Autodesk Inventor part; units mm, degrees
ref_plane "YZ Plane" through (0, 0, 0) normal (1, 0, 0) x (0, 1, 0)
ref_plane "XZ Plane" through (0, 0, 0) normal (0, 1, 0) x (-1, 0, 0)
ref_plane "XY Plane" through (0, 0, 0) normal (0, 0, 1) x (1, 0, 0)
sketch "Sketch1" plane through (0, 0, 0) normal (0, 0, 1) x (1, 0, 0)
  line L0 (5.9771, 0) -> (28.2021, 0)
  line L1 (28.2021, 0) -> (28.2021, 3.175)
  line L2 (28.2021, 3.175) -> (5.9771, 3.175)
  line L3 (2.8021, 6.35) -> (2.8021, 25.4)
  line L4 (5.9771, 28.575) -> (28.2021, 28.575)
  line L5 (28.2021, 28.575) -> (28.2021, 31.75)
  line L6 (28.2021, 31.75) -> (5.9771, 31.75)
  line L7 (-0.3729, 25.4) -> (-0.3729, 6.35)
  arc A0 (5.9771, 28.575) -> (2.8021, 25.4) centre (5.9771, 25.4) ccw
  arc A1 (2.8021, 6.35) -> (5.9771, 3.175) centre (5.9771, 6.35) ccw
  arc A2 (5.9771, 31.75) -> (-0.3729, 25.4) centre (5.9771, 25.4) ccw
  arc A3 (-0.3729, 6.35) -> (5.9771, 0) centre (5.9771, 6.35) ccw
  point P0 (0, 0)
  point P1 (-0.3729, 0)
  point P2 (2.8021, 3.175)
  point P3 (2.8021, 28.575)
  dimension "d0" = 28.575
  dimension "d1" = 3.175
  dimension "d2" = 25.4
  dimension "d3" = 25.4
  dimension "d4" = 3.175
  dimension "d5" = 3.175
  dimension "d6" = 6.35
extrude "Extrusion1" add sketch "Sketch1" against normal blind 889
sketch "Sketch2" plane through (-0.3729, 6.35, 0) normal (-1, 0, 0) x (0, 0, 1)
  line L0 (0, 19.05) -> (-889, 19.05)
  line L1 (-228.6, 0) -> (-228.6, 7.9375)
  arc A0 (-228.6, 11.1125) -> (-228.6, 7.9375) centre (-228.6, 9.525) ccw
  line L2 (-228.6, 11.1125) -> (-228.6, 19.05)
  line L3 (-228.6, 19.05) -> (-889, 19.05)
  line L4 (-889, 0) -> (-889, 19.05)
  line L5 (-889, 0) -> (-228.6, 0)
  circle A1 centre (-552.45, 11.43) radius 4.826
  circle A2 centre (-501.65, 11.43) radius 4.826
  circle A3 centre (-387.35, 11.43) radius 4.826
  circle A4 centre (-336.55, 11.43) radius 4.826
  circle A5 centre (-444.5, 7.62) radius 4.826
  circle A6 centre (-730.25, 11.43) radius 4.826
  circle A7 centre (-781.05, 11.43) radius 4.826
  line L6 (0, 25.4) -> (-889, 25.4) construction
  circle A8 centre (-133.35, 11.43) radius 4.826
  circle A9 centre (-82.55, 11.43) radius 4.826
  point P0 (0, -6.35)
  point P1 (-254, 0.852)
  dimension "d10" = 7.62
  dimension "d11" = 3.81
  dimension "d14" = 254
hole "Hole1" at (-0.3729, 17.78, -781.05) at (-0.3729, 17.78, -730.25) at (-0.3729, 17.78, -552.45) at (-0.3729, 17.78, -501.65) at (-0.3729, 13.97, -444.5) at (-0.3729, 17.78, -387.35) at (-0.3729, 17.78, -336.55) at (-0.3729, 17.78, -133.35) at (-0.3729, 17.78, -82.55) direction (1, 0, 0) diameter 9.652 end through all
hole "Hole2" at (-0.3729, 15.875, -228.6) direction (1, 0, 0) diameter 3.175 end through all
sketch "Sketch3" plane through (5.9771, 31.75, 0) normal (0, 1, 0) x (1, 0, 0)
  line L0 (22.225, 889) -> (0, 889)
  line L1 (22.225, 0) -> (22.225, 889)
  point P0 (-5.9771, 0)
  point P1 (9.525, 876.3)
  dimension "d34" = 12.7
  dimension "d35" = 12.7
hole "Hole3" at (15.5021, 31.75, -876.3) direction (0, -1, 0) diameter 6.5278 end through all
pattern_linear "Rectangular Pattern1" count 35 spacing 25.4 along (0, 0, 1) of "Hole3"
sketch "Sketch4" plane through (5.9771, 31.75, 0) normal (0, 1, 0) x (1, 0, 0)
  circle A0 centre (9.525, 12.7) radius 3.2639
  circle A1 centre (9.525, 38.1) radius 3.2639
  circle A2 centre (9.525, 63.5) radius 3.2639
  circle A3 centre (9.525, 88.9) radius 3.2639
  circle A4 centre (9.525, 114.3) radius 3.2639
  circle A5 centre (9.525, 139.7) radius 3.2639
  circle A6 centre (9.525, 165.1) radius 3.2639
  circle A7 centre (9.525, 190.5) radius 3.2639
  line L0 (22.225, 0) -> (-13.6032, 0)
  line L1 (-13.6032, 0) -> (-13.6032, 508)
  line L2 (-13.6032, 508) -> (22.225, 508)
  line L3 (22.225, 508) -> (22.225, 0)
  point P0 (-5.9771, 0)
  dimension "d46" = 508
extrude "Extrusion2" cut sketch "Sketch4" against normal blind 38.1
properties part number "chassis 15 inch"
Could you check a few things on this model? Use its own coordinates, in mm. A direction names the side the tool comes from. Give positions to 0.01 mm unless a question says otherwise; leave off trailing zeros. Order: outer loops, then holes, each group sorted by start corner. A loop starts at its lowest first (then second) coordinate and runs counter-clockwise, first axis right, second up.
1. Suppose I cut it at B-B (z = -800.1). List the corners of the cut face in (x, y) for me (3 decimals), plus the area to 3 significant figures.
2. Will these pins go through, and if not, where does the flat tip stop? P1, Ø8.5, axis at x = 15.5, z = -774.7, coming from the -Y side; P2, Ø1.5, axis at y = 27, z = -690.5, coming from the -X side.
3. Suppose I cut it at A-A (y = 17.78). List the corners of the cut face in (x, z) for me, plus the area to 3 significant figures.
4. We'd pull the mould along Z, two halves only. Please class faces 1 (the cylindrical face through (14.522, 1.565, -873.187)), 2 (the cylindrical face through (1.44, 1.91, -695.83)): pulls with the +Z half, pulls with the -Z half, needs draft (parallel to the pull), parting line crosses it, or undercut.
5. Suppose I cut it at C-C (z = -655.5). List the corners of the cut face in (x, y) for me (3 decimals).
6. I need wall thicknesses on L1, parallel to Y at x = 12, z = -834 (3 decimals); L2, parallel to Y at x = 5.5, z = -737; L3, parallel to X at y = 20, z = -799. Which ranges of each line are inside material? Lowest first, please.
7. For faces 3 (the flat face through (19, 28.575, -696)), 4 (the flat face through (19, 0, -696)), which set-ups out of +Z, -Z, +X, -X, +Y, -Y let a thin tool reach every point of the face, with its end or its side?
Solved:
1. outline: (-0.373, 6.35) arc R6.35 ccw to (5.977, 0) - (12.238, 0) - (12.238, 3.175) - (5.977, 3.175) arc R3.175 cw to (2.802, 6.35) - (2.802, 25.4) arc R3.175 cw to (5.977, 28.575) - (12.238, 28.575) - (12.238, 31.75) - (5.977, 31.75) arc R6.35 ccw to (-0.373, 25.4) - close; (18.766, 0) - (28.202, 0) - (28.202, 3.175) - (18.766, 3.175) - close; (18.766, 28.575) - (28.202, 28.575) - (28.202, 31.75) - (18.766, 31.75) - close
1. area: 208 mm2
2. P1: stops at y = 0
2. P2: stops at x = -0.32
3. outline: (-0.37, -889) - (2.8, -889) - (2.8, -785.88) - (-0.37, -785.88) - close; (-0.37, -776.22) - (2.8, -776.22) - (2.8, -735.08) - (-0.37, -735.08) - close; (-0.37, -725.42) - (2.8, -725.42) - (2.8, -557.28) - (-0.37, -557.28) - close; (-0.37, -547.62) - (2.8, -547.62) - (2.8, -508) - (-0.37, -508) - close
3. area: 1,120 mm2
4. face 1: undercut
4. face 2: needs draft
5. outline: (-0.373, 6.35) arc R6.35 ccw to (5.977, 0) - (28.202, 0) - (28.202, 3.175) - (5.977, 3.175) arc R3.175 cw to (2.802, 6.35) - (2.802, 25.4) arc R3.175 cw to (5.977, 28.575) - (28.202, 28.575) - (28.202, 31.75) - (5.977, 31.75) arc R6.35 ccw to (-0.373, 25.4) - close
6. L1: y = 0 to 3.175, 28.575 to 31.75
6. L2: y = 0.02 to 3.21, 28.54 to 31.73
6. L3: x = -0.37 to 2.8
7. face 3: +Z, -Z, +X
7. face 4: +Z, -Z, +X, -X, -Y
